Input: part model. Units: mm. Frame: model coordinates. Face numbers are marked on the shaded views. Coordinates: 2 decimals unless noted, no trailing zeros. Loops run counter-clockwise (first coordinate to the right, second up) from the corner with the lowest first, then second, coordinate; pieces in that order, holes last. Notation, with made-up numbers: (63.5, -15.5) -> (96.5, -15.5) arc R15 ccw to (96.5, -11.5) -> close; hole circle Ø9 at (2, -13). An arc over 180 degrees is marked (long way). Answer as a JSON object with one key per item and string values.
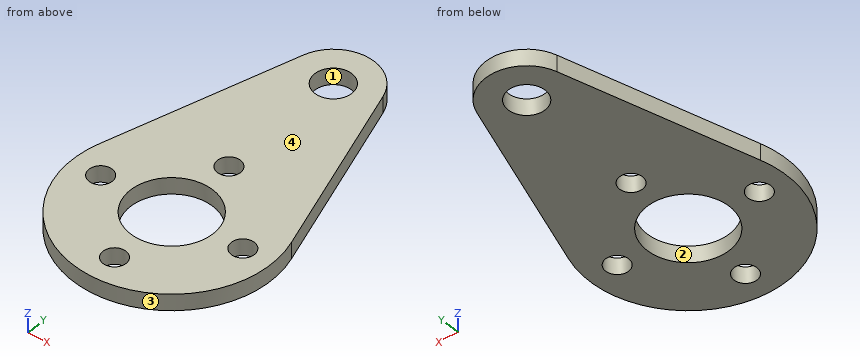
Autodesk Inventor part; units mm, degrees
ref_plane "YZ Plane" through (0, 0, 0) normal (1, 0, 0) x (0, 1, 0)
ref_plane "XZ Plane" through (0, 0, 0) normal (0, 1, 0) x (-1, 0, 0)
ref_plane "XY Plane" through (0, 0, 0) normal (0, 0, 1) x (1, 0, 0)
sketch "スケッチ1" plane through (0, 0, 0) normal (0, 0, 1) x (1, 0, 0)
  circle A0 centre (0, 0) radius 5
  arc A1 (-11.4782, 3.5) -> (11.4782, 3.5) centre (0, 0) ccw
  arc A2 (4.7826, 25.4583) -> (-4.7826, 25.4583) centre (0, 24) ccw
  line L0 (-4.7826, 25.4583) -> (-11.4782, 3.5)
  line L1 (4.7826, 25.4583) -> (11.4782, 3.5)
  dimension "d0" = 10
  dimension "d1" = 24
  dimension "d2" = 10
  dimension "d3" = 24
extrude "押し出し1" add sketch "スケッチ1" along normal blind 2
sketch "スケッチ2" plane through (0, 0, 2) normal (0, 0, 1) x (1, 0, 0)
  line L0 (0, 0) -> (12, 0) construction
  arc A0 (-11.4782, 3.5) -> (11.4782, 3.5) centre (0, 0) ccw
  line L1 (0, 0) -> (0, 12) construction
  line L2 (0, 0) -> (-12, 0) construction
  line L3 (0, 0) -> (0, -12) construction
  point P0 (8.5, 0)
  point P1 (0, 8.5)
  point P2 (-8.5, 0)
  point P3 (0, -8.5)
  dimension "d6" = 8.5
  dimension "d9" = 360
hole "穴1" at (8.5, 0, 2) at (0, 8.5, 2) at (-8.5, 0, 2) at (0, -8.5, 2) direction (0, 0, -1) diameter 2.8 end through all
sketch "スケッチ3" plane through (0, 0, 2) normal (0, 0, 1) x (1, 0, 0)
  arc A0 (4.7826, 25.4583) -> (-4.7826, 25.4583) centre (0, 24) ccw
  point P0 (0, 0)
hole "穴2" at (0, 24, 2) direction (0, 0, -1) diameter 4.5 end through all
properties part number "lever"
1. Line query: line 1 along Y through (x, z) = (0, 0.1); line 2 along Y through (x, z) = (-1.25, 0.1); line 3 along X through (y, z) = (8, 0.4). Output: solid intervals per line, ascending.
Reply:
{"line 1": "y = -12 to -9.9, -7.1 to -5, 5 to 7.1, 9.9 to 21.75, 26.25 to 29", "line 2": "y = -11.93 to -9.13, -7.87 to -4.84, 4.84 to 7.87, 9.13 to 22.13, 25.87 to 28.84", "line 3": "x = -10.11 to -1.31, 1.31 to 10.11"}
2. Section query C-C (y = 0). Return loops of the section in (x, z), plus the area to 3 significant figures.
Reply:
{"outline": "(-12, 0) -> (-9.9, 0) -> (-9.9, 2) -> (-12, 2) -> close; (-7.1, 0) -> (-5, 0) -> (-5, 2) -> (-7.1, 2) -> close; (5, 0) -> (7.1, 0) -> (7.1, 2) -> (5, 2) -> close; (9.9, 0) -> (12, 0) -> (12, 2) -> (9.9, 2) -> close", "area": "16.8 mm2"}
3. Section query B-B (x = 8.5). Return loops of the section in (y, z), plus the area to 3 significant figures.
Reply:
{"outline": "(-8.47, 0) -> (-1.4, 0) -> (-1.4, 2) -> (-8.47, 2) -> close; (1.4, 0) -> (13.27, 0) -> (13.27, 2) -> (1.4, 2) -> close", "area": "37.9 mm2"}
4. Section query A-A (z = 1.65). Return loops of the section in (x, y).
Reply:
{"outline": "(-11.48, 3.5) arc R12 ccw (long way) to (11.48, 3.5) -> (4.78, 25.46) arc R5 ccw to (-4.78, 25.46) -> close; hole circle Ø2.8 at (-8.5, 0); hole circle Ø10 at (0, 0); hole circle Ø4.5 at (0, 24); hole circle Ø2.8 at (0, -8.5); hole circle Ø2.8 at (0, 8.5); hole circle Ø2.8 at (8.5, 0)"}
5. Pin query (flat end, axial travel): P1, Ø3.5, axis at x = 0, y = 24, coming from the +Z side; P2, Ø1, axis at x = 1, z = 0.5, coming from the +Y side. Return the tip coordinate at first contact, or that it passes through.
Reply:
{"P1": "passes through", "P2": "stops at y = 28.97"}
6. Section query D-D (x = 0). Return loops of the section in (y, z).
Reply:
{"outline": "(-12, 0) -> (-9.9, 0) -> (-9.9, 2) -> (-12, 2) -> close; (-7.1, 0) -> (-5, 0) -> (-5, 2) -> (-7.1, 2) -> close; (5, 0) -> (7.1, 0) -> (7.1, 2) -> (5, 2) -> close; (9.9, 0) -> (21.75, 0) -> (21.75, 2) -> (9.9, 2) -> close; (26.25, 0) -> (29, 0) -> (29, 2) -> (26.25, 2) -> close"}
7. Mould query, pull axis Y, two halves, no side actions, for the marked faces 1, 2, 3 and 4. Classes: pulls with the +Y half, pulls with the -Y half, needs draft (parallel to the pull), parting line crosses it, or undercut.
Reply:
{"face 1": "undercut", "face 2": "undercut", "face 3": "parting line crosses it", "face 4": "needs draft"}
